Read the model definition and answer for the solid it produces. Units are mm, in the model's axes. Coordinates: 2 decimals unless noted, no trailing zeros. Answer in a Markdown table with one row per item. Add a question column.
Item 1: For a pull along X with two mould halves and no side action, classify faces 1 (the face through (-16.132, -38.945, -51.227)), 2 (the face through (57.31, -38.29, 12.73)) as +X half, -X half, draft (parallel to the pull), parting line (faces both ways), or undercut.
Item 2: Given pin 1 Ø1.5 at (y, z) = (-6.5, -8) entering from -X; pin 2 Ø12 at (y, z) = (-33, -23.5) entering from -X; pin 3 Ø1 at (x, z) = (-31.5, -31.5) entering from -Y, each flat-ended and moving along its own axis, determine where each tip first touches the part or whether it passes through.
Item 3: Straight lines are drawn through the part: line 1 (X direction, y = -8, z = -3); line 2 (Y direction, x = -40, z = -44); line 3 (X direction, y = -22.5, z = -19.5). For each, find the intervals that lie inside material, in ascending order. Write a range as from..to.
```python
from build123d import *

# Parameters (mm, degrees)
CROQUIS3_R                 = 0.15
SALIENTE_EXTRUIR1_DEPTH    = 1
MATRIZC1_COUNT             = 8
CORTAR_EXTRUIR1_DEPTH      = 3.5
CORTAR_EXTRUIR1_DEPTH_BACK = 3.5


with BuildPart() as part:
    # Croquis1 → Revolución1 (revolve)
    with BuildSketch(Plane(origin=(0, 0, 0), x_dir=(0, 0, -1), z_dir=(1, 0, 0)), mode=Mode.PRIVATE) as revoluci_n1_sk:
        with BuildLine():
            Line((-53.706749403, -38.00205598), (-53.706749403, -39.862857986))
            ThreePointArc((-53.706749403, -39.862857986), (-66.128903849, -50.946483139), (-82.75, -50))
            Line((-82.75, -50), (-82.75, -45.913633918))
            ThreePointArc((-82.75, -45.913633918), (-81.749843887, -45.255213155), (-80.577052932, -45.496856538))
            ThreePointArc((-80.577052932, -45.496856538), (-68.28580191, -46.394407616), (-58.706749403, -38.640556786))
            Line((-58.706749403, -38.640556786), (-58.706749403, -37.948984749))
            ThreePointArc((-58.706749403, -37.948984749), (-56.396956017, -26.15017016), (-50.225083134, -15.832459353))
            ThreePointArc((-50.225083134, -15.832459353), (-27.121918445, -0.727624897), (-0.119641632, 4.998568383))
            Line((-0.119641632, 4.998568383), (0, 4.998568383))
            Line((0, 4.998568383), (0, 0))
            ThreePointArc((0, 0), (-25.090629498, -5.29813609), (-46.590589513, -19.275319426))
            ThreePointArc((-46.590589513, -19.275319426), (-51.761100349, -28.025963964), (-53.706749403, -38.00205598))
        make_face()
    revolve(revoluci_n1_sk.sketch.rotate(Axis((0, 0, 0), (0, 1, 0)), 180), axis=Axis((0, 0, 0), (0, 1, 0)))

    # Croquis3 → Saliente-Extruir1 (add)
    with BuildSketch(Plane.XY):
        with BuildLine():
            Line((-82.669777011, -47.619178632), (-82.96122925, -47.619178632))
            ThreePointArc((-82.96122925, -47.619178632), (-83.138005946, -47.692401937), (-83.21122925, -47.869178632))
            Line((-83.21122925, -47.869178632), (-83.21122925, -47.903618104))
            ThreePointArc((-83.21122925, -47.903618104), (-83.138005946, -48.080394799), (-82.96122925, -48.153618104))
            Line((-82.96122925, -48.153618104), (-82.669777011, -48.153618104))
            Line((-82.669777011, -48.153618104), (-82.669777011, -47.619178632))
        make_face()
        with Locations((-82.953032146, -47.876545308)):
            Circle(CROQUIS3_R, mode=Mode.SUBTRACT)
    saliente_extruir1 = extrude(amount=SALIENTE_EXTRUIR1_DEPTH)

    # MatrizC1: Saliente-Extruir1 ×8 about axis
    matrizc1_axis = Axis((0, 0, 0), (0, 1, 0))
    for i in range(1, MATRIZC1_COUNT):
        add(saliente_extruir1.rotate(matrizc1_axis, i * 360 / MATRIZC1_COUNT))

    # Croquis4 → Cortar-Extruir1 (cut, two sides: drawn at the far end of the back side and taken through both)
    with BuildSketch(Plane(origin=(0, 0, 0), x_dir=(0, 0, -1), z_dir=(1, 0, 0)).offset(-CORTAR_EXTRUIR1_DEPTH_BACK)):
        with BuildLine():
            Line((-13.463399876, -1.873922968), (14.527518877, -1.873922968))
            ThreePointArc((14.527518877, -1.873922968), (0.532059501, 0.452935275), (-13.463399876, -1.873922968))
        make_face()
    extrude(amount=CORTAR_EXTRUIR1_DEPTH + CORTAR_EXTRUIR1_DEPTH_BACK, mode=Mode.SUBTRACT)


solid = part.part
```
Results below:
| question | item | result |
|---|---|---|
| 1 | face 1 | undercut |
| 1 | face 2 | parting line |
| 2 | pin 1 | stops at x = -38.63 |
| 2 | pin 2 | stops at x = -55.74 |
| 2 | pin 3 | stops at y = -17.85 |
| 3 | line 1 | x = -40.45..-30.72, 30.72..40.45 |
| 3 | line 2 | y = -47.2..-39.86 |
| 3 | line 3 | x = -51.16..-44.93, 44.93..51.16 |
